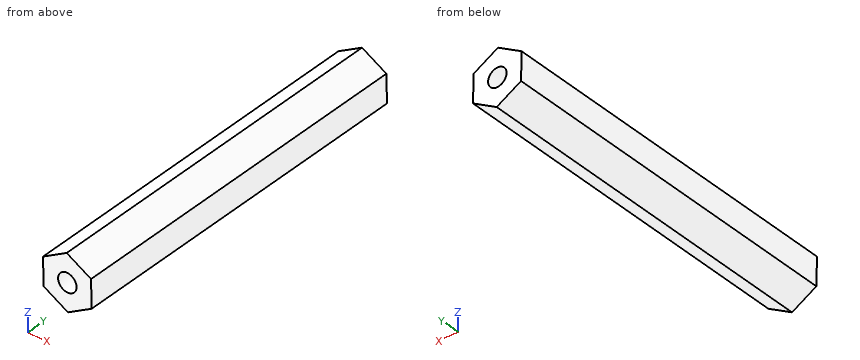
from build123d import *

# Parameters (mm, degrees)
BOSS_EXTRUDE1_DEPTH = 47.5
SKETCH1_3_R         = 2.5
CUT_EXTRUDE1_DEPTH  = 52


with BuildPart() as part:
    # Sketch1 → Boss-Extrude1 (new, symmetric)
    with BuildSketch(Plane(origin=(0, 0, 0), x_dir=(1, 0, 0), z_dir=(0, 1, 0))):
        Polygon((6.584646409, 3.602188918), (0.172736092, 7.503565524), (-6.411910317, 3.901376606), (-6.584646409, -3.602188918), (-0.172736092, -7.503565524), (6.411910317, -3.901376606), align=None)
    extrude(amount=BOSS_EXTRUDE1_DEPTH, both=True)

    # Sketch1_3 → Cut-Extrude1 (cut, symmetric)
    with BuildSketch(Plane(origin=(0, 0, 0), x_dir=(1, 0, 0), z_dir=(0, 1, 0))):
        with Locations(Location((0, 0, 0), (0, 0, 270))):
            Circle(SKETCH1_3_R)
    extrude(amount=CUT_EXTRUDE1_DEPTH, both=True, mode=Mode.SUBTRACT)


solid = part.part
Input: part model. Units: mm. Frame: model coordinates. Coordinates: 2 decimals unless noted, no trailing zeros. Write each loop counter-clockwise with the first axis right and the second up, starting at its lowest first coordinate (ties: lowest second). Pieces come first, ordered by that corner, then holes. Notation, with made-up numbers: M 1.5,-22.5 L 51.5,-22.5 A9 ccw 51.5,-6.5 Z; hole C 57,30.25 d10. An arc over 180 degrees is marked long. Answer as a JSON object with one key per item and string values. Group by question number.
(1) Section C-C on x = 5.5. Output: boundary loops of the cut face in (y, z), plus the area to 3 significant figures.
(2) Section A-A on y = 36. Output: boundary loops of the cut face in (x, z), plus the area to 3 significant figures.
(3) Section B-B on z = 0. Output: boundary loops of the cut face in (x, y), plus the area to 3 significant figures.
(4) Section D-D on z = -6. Output: boundary loops of the cut face in (x, y).
(5) Contact query for flat-ended pins moving along their axis: P1, Ø4, axis at y = -26, z = -4.5, coming from the -X side; P2, Ø5, axis at x = -3, y = 4, coming from the +Z side; P3, Ø1, axis at y = 27.5, z = 1, coming from the -X side. Output: stop coordinate, or through.
(6) Ray query, line 1 along X through (y, z) = (38.5, 2); line 2 along Z through (x, y) = (-1.5, 5.5); line 3 along X through (y, z) = (-11.5, 0). Return the intervals inside material, ascending. Write a range as [from, to].
Result set:
{
 "1": {"outline": "M -47.5,-4.26 L 47.5,-4.26 L 47.5,4.4 L -47.5,4.4 Z", "area": "823 mm2"},
 "2": {"outline": "M -6.58,3.6 L -6.41,-3.9 L 0.17,-7.5 L 6.58,-3.6 L 6.41,3.9 L -0.17,7.5 Z; hole C 0,0 d5", "area": "127 mm2"},
 "3": {"outline": "M -6.5,-47.5 L -2.5,-47.5 L -2.5,47.5 L -6.5,47.5 Z; M 2.5,-47.5 L 6.5,-47.5 L 6.5,47.5 L 2.5,47.5 Z", "area": "760 mm2"},
 "4": {"outline": "M -2.58,-47.5 L 2.64,-47.5 L 2.64,47.5 L -2.58,47.5 Z"},
 "5": {"P1": "stops at x = -6.44", "P2": "stops at z = 7.3", "P3": "stops at x = -6.54"},
 "6": {"line 1": "x = [-6.55, -1.5], [1.5, 6.46]", "line 2": "z = [-6.59, -2], [2, 6.7]", "line 3": "x = [-6.5, -2.5], [2.5, 6.5]"}
}
